For this review, take the finished solid that the model builds, in its own axes (mm). Coordinates: 2 decimals unless noted, no trailing zeros. Write each loop counter-clockwise with the first axis right and the second up, starting at its lowest first coordinate (ties: lowest second). Pieces come first, ordered by that corner, then holes. Notation, with made-up numbers: (62.25, 10.25) -> (94.25, 10.25) arc R30 ccw to (94.25, 41.25) -> close; hole circle Ø7 at (34, 53). An arc over 180 degrees is marked (long way). Put each result on its own line as item: value. Start each with the question number.
Item 1: Consider section B-B on x = -38.5. Give the boundary of the cut face in (y, z).
Item 2: Consider section C-C on y = 65. Give the boundary of the cut face in (x, z), and give its area (3 significant figures).
Item 3: To check wall thickness, follow L1, parallel to Y at x = -39.5, z = 4.5; L2, parallel to Y at x = -122, z = 1.8; L3, parallel to Y at x = -122.5, z = 2.4. State the ranges of each line that lie inside material, in increasing order.
Item 4: Insertion check: P1, Ø1.5, axis at x = -141.5, z = 3.5, coming from the +Y side; P2, Ø1.5, axis at y = 63, z = 1.5, coming from the +X side; P3, Ø1.5, axis at x = -116.5, z = 2, coming from the +Y side. Each pin has a flat end and moves straight along its axis. Give the tip position at first contact, or say it passes through.
Autodesk Inventor part; units mm, degrees
ref_plane "YZ Plane" through (0, 0, 0) normal (1, 0, 0) x (0, 1, 0)
ref_plane "XZ Plane" through (0, 0, 0) normal (0, 1, 0) x (-1, 0, 0)
ref_plane "XY Plane" through (0, 0, 0) normal (0, 0, 1) x (1, 0, 0)
sketch "Sketch1" plane through (0, 0, 0) normal (0, 0, 1) x (1, 0, 0)
  line L0 (0, 0) -> (0, 92)
  line L1 (0, 92) -> (-70, 92)
  line L2 (-70, 92) -> (-161.8477, 0)
  line L3 (-161.8477, 0) -> (0, 0)
  dimension "d1" = 70
  dimension "d2" = 130
  dimension "d7" = 92
extrude "Extrusion1" add sketch "Sketch1" along normal blind 5
sketch "Sketch2" plane through (0, 0, 5) normal (0, 0, 1) x (1, 0, 0)
  line L0 (-70, 92) -> (-161.8477, 0)
  line L1 (-143.5135, 18.3646) -> (-139.9043, 14.7614)
  line L2 (-139.9043, 14.7614) -> (-121.4641, 33.2321)
  line L3 (-121.4641, 33.2321) -> (-125.0733, 36.8354)
  line L4 (-106.7744, 55.1646) -> (-103.1652, 51.5614)
  line L5 (-103.1652, 51.5614) -> (-84.725, 70.0321)
  line L6 (-84.725, 70.0321) -> (-88.3342, 73.6354)
  line L7 (-123.2687, 35.0338) -> (-104.9698, 53.363) construction
  line L8 (-114.1192, 44.1984) -> (-115.9239, 46)
  line L9 (-161.8477, 0) -> (0, 0)
  line L10 (-129.5282, 0) -> (-97.0586, 0)
  line L11 (-97.0586, 0) -> (-97.0586, 5.1)
  line L12 (-97.0586, 5.1) -> (-129.5282, 5.1)
  line L13 (-129.5282, 5.1) -> (-129.5282, 0)
  line L14 (-64.7891, 0) -> (-32.3195, 0)
  line L15 (-32.3195, 0) -> (-32.3195, 5.1)
  line L16 (-32.3195, 5.1) -> (-64.7891, 5.1)
  line L17 (-64.7891, 5.1) -> (-64.7891, 0)
  line L18 (0, 18.35) -> (-5.1, 18.35)
  line L19 (-5.1, 18.35) -> (-5.1, 36.85)
  line L20 (-5.1, 36.85) -> (0, 36.85)
  line L21 (0, 36.85) -> (0, 18.35)
  line L22 (0, 55.15) -> (-5.1, 55.15)
  line L23 (-5.1, 55.15) -> (-5.1, 73.65)
  line L24 (-5.1, 73.65) -> (0, 73.65)
  line L25 (0, 73.65) -> (0, 55.15)
  line L26 (0, 92) -> (-70, 92)
  line L27 (-46.7167, 92) -> (-23.2833, 92)
  line L28 (-23.2833, 92) -> (-23.2833, 86.9)
  line L29 (-23.2833, 86.9) -> (-46.7167, 86.9)
  line L30 (-46.7167, 86.9) -> (-46.7167, 92)
  line L31 (0, 0) -> (0, 92)
  line L32 (-2.55, 36.85) -> (-2.55, 55.15) construction
  line L33 (-64.7891, 2.55) -> (-97.0586, 2.55) construction
  point P0 (-35, 86.9)
  point P1 (-35, 92)
  point P2 (-80.9239, 2.55)
  point P3 (-80.9239, 0)
  point P4 (-2.55, 46)
  point P5 (0, 46)
  point P6 (-35, 92)
  dimension "d8" = 130
  dimension "d9" = 26.1
  dimension "d10" = 25.9
  dimension "d13" = 5.1
  dimension "d14" = 70
  dimension "d15" = 92
  dimension "d16" = 161.8477
  dimension "d17" = 32.2695
  dimension "d18" = 32.4695
  dimension "d19" = 18.3
  dimension "d20" = 18.5
  dimension "d21" = 23.4333
extrude "Extrusion2" cut sketch "Sketch2" against normal blind 10 contours L6 L5 L4 L0 | L26 L28 L29 L30 | L3 L2 L1 L0 | L25 L22 L23 L24 | L21 L18 L19 L20 | L13 L12 L11 L9 | L17 L16 L15 L9
sketch "Sketch3" plane through (0, 0, 5) normal (0, 0, 1) x (1, 0, 0)
  line L0 (-5.1, 36.85) -> (0, 36.85)
  line L1 (0, 36.85) -> (0, 55.15)
  line L2 (0, 55.15) -> (-5.1, 55.15)
  line L3 (-5.1, 55.15) -> (-5.1, 73.65)
  line L4 (-5.1, 73.65) -> (0, 73.65)
  line L5 (0, 73.65) -> (0, 92)
  line L6 (0, 92) -> (-23.2833, 92)
  line L7 (-23.2833, 92) -> (-23.2833, 86.9)
  line L8 (-23.2833, 86.9) -> (-46.7167, 86.9)
  line L9 (-46.7167, 86.9) -> (-46.7167, 92)
  line L10 (-46.7167, 92) -> (-70, 92)
  line L11 (-70, 92) -> (-88.3342, 73.6354)
  line L12 (-88.3342, 73.6354) -> (-84.725, 70.0321)
  line L13 (-84.725, 70.0321) -> (-103.1652, 51.5614)
  line L14 (-103.1652, 51.5614) -> (-106.7744, 55.1646)
  line L15 (-106.7744, 55.1646) -> (-125.0733, 36.8354)
  line L16 (-125.0733, 36.8354) -> (-121.4641, 33.2321)
  line L17 (-121.4641, 33.2321) -> (-139.9043, 14.7614)
  line L18 (-139.9043, 14.7614) -> (-143.5135, 18.3646)
  line L19 (-143.5135, 18.3646) -> (-161.8477, 0)
  line L20 (-161.8477, 0) -> (-129.5282, 0)
  line L21 (-129.5282, 0) -> (-129.5282, 5.1)
  line L22 (-129.5282, 5.1) -> (-97.0586, 5.1)
  line L23 (-97.0586, 5.1) -> (-97.0586, 0)
  line L24 (-97.0586, 0) -> (-64.7891, 0)
  line L25 (-64.7891, 0) -> (-64.7891, 5.1)
  line L26 (-64.7891, 5.1) -> (-32.3195, 5.1)
  line L27 (-32.3195, 5.1) -> (-32.3195, 0)
  line L28 (-32.3195, 0) -> (0, 0)
  line L29 (0, 0) -> (0, 18.35)
  line L30 (0, 18.35) -> (-5.1, 18.35)
  line L31 (-5.1, 18.35) -> (-5.1, 36.85)
  line L32 (-132.1444, 36.8295) -> (-106.7803, 62.2357)
  line L33 (-106.7803, 62.2357) -> (-103.171, 58.6324)
  line L34 (-103.171, 58.6324) -> (-91.796, 70.0263)
  line L35 (-91.796, 70.0263) -> (-95.4053, 73.6295)
  line L36 (-95.4053, 73.6295) -> (-72.0735, 97)
  line L37 (-72.0735, 97) -> (-41.7167, 97)
  line L38 (-41.7167, 97) -> (-41.7167, 91.9)
  line L39 (-41.7167, 91.9) -> (-28.2833, 91.9)
  line L40 (-28.2833, 91.9) -> (-28.2833, 97)
  line L41 (-28.2833, 97) -> (5, 97)
  line L42 (5, 97) -> (5, 68.65)
  line L43 (5, 68.65) -> (-0.1, 68.65)
  line L44 (-0.1, 68.65) -> (-0.1, 60.15)
  line L45 (-0.1, 60.15) -> (5, 60.15)
  line L46 (5, 60.15) -> (5, 31.85)
  line L47 (5, 31.85) -> (-0.1, 31.85)
  line L48 (-0.1, 31.85) -> (-0.1, 23.35)
  line L49 (-0.1, 23.35) -> (5, 23.35)
  line L50 (5, 23.35) -> (5, -5)
  line L51 (5, -5) -> (-37.3195, -5)
  line L52 (-37.3195, -5) -> (-37.3195, 0.1)
  line L53 (-37.3195, 0.1) -> (-59.7891, 0.1)
  line L54 (-59.7891, 0.1) -> (-59.7891, -5)
  line L55 (-59.7891, -5) -> (-102.0586, -5)
  line L56 (-102.0586, -5) -> (-102.0586, 0.1)
  line L57 (-102.0586, 0.1) -> (-124.5282, 0.1)
  line L58 (-124.5282, 0.1) -> (-124.5282, -5)
  line L59 (-124.5282, -5) -> (-173.9046, -5)
  line L60 (-173.9046, -5) -> (-143.5193, 25.4357)
  line L61 (-143.5193, 25.4357) -> (-139.9101, 21.8324)
  line L62 (-139.9101, 21.8324) -> (-128.5351, 33.2263)
  line L63 (-128.5351, 33.2263) -> (-132.1444, 36.8295)
  line L64 (-143.5135, 18.3646) -> (-147.0519, 21.8972)
  line L65 (-161.8477, 0) -> (-168.9129, 0)
  line L66 (-125.0733, 36.8354) -> (-128.6118, 40.368)
  line L67 (-106.7744, 55.1646) -> (-110.3129, 58.6972)
  line L68 (-103.171, 58.6324) -> (-106.7744, 55.1646)
  line L69 (-91.796, 70.0263) -> (-88.3342, 73.6354)
  line L70 (-88.3342, 73.6354) -> (-91.8727, 77.168)
  line L71 (-70, 92) -> (-77.0652, 92)
  line L72 (-139.9101, 21.8324) -> (-143.5135, 18.3646)
  line L73 (-125.0733, 36.8354) -> (-128.5351, 33.2263)
  line L74 (-143.5135, 18.3646) -> (-161.8477, 0)
  line L75 (-161.8477, 0) -> (-165.3862, 3.5326)
  dimension "d22" = 5
extrude "Extrusion3" [suppressed]
sketch "Sketch4" plane through (0, 0, 5) normal (0, 0, 1) x (1, 0, 0)
  line L0 (-5.1, 36.85) -> (0, 36.85)
  line L1 (0, 36.85) -> (0, 55.15)
  line L2 (0, 55.15) -> (-5.1, 55.15)
  line L3 (-5.1, 55.15) -> (-5.1, 73.65)
  line L4 (-5.1, 73.65) -> (0, 73.65)
  line L5 (0, 73.65) -> (0, 92)
  line L6 (0, 92) -> (-23.2833, 92)
  line L7 (-23.2833, 92) -> (-23.2833, 86.9)
  line L8 (-23.2833, 86.9) -> (-46.7167, 86.9)
  line L9 (-46.7167, 86.9) -> (-46.7167, 92)
  line L10 (-46.7167, 92) -> (-70, 92)
  line L11 (-70, 92) -> (-88.3342, 73.6354)
  line L12 (-88.3342, 73.6354) -> (-84.725, 70.0321)
  line L13 (-84.725, 70.0321) -> (-103.1652, 51.5614)
  line L14 (-103.1652, 51.5614) -> (-106.7744, 55.1646)
  line L15 (-106.7744, 55.1646) -> (-125.0733, 36.8354)
  line L16 (-125.0733, 36.8354) -> (-121.4641, 33.2321)
  line L17 (-121.4641, 33.2321) -> (-139.9043, 14.7614)
  line L18 (-139.9043, 14.7614) -> (-143.5135, 18.3646)
  line L19 (-143.5135, 18.3646) -> (-161.8477, 0)
  line L20 (-161.8477, 0) -> (-129.5282, 0)
  line L21 (-129.5282, 0) -> (-129.5282, 5.1)
  line L22 (-129.5282, 5.1) -> (-97.0586, 5.1)
  line L23 (-97.0586, 5.1) -> (-97.0586, 0)
  line L24 (-97.0586, 0) -> (-64.7891, 0)
  line L25 (-64.7891, 0) -> (-64.7891, 5.1)
  line L26 (-64.7891, 5.1) -> (-32.3195, 5.1)
  line L27 (-32.3195, 5.1) -> (-32.3195, 0)
  line L28 (-32.3195, 0) -> (0, 0)
  line L29 (0, 0) -> (0, 18.35)
  line L30 (0, 18.35) -> (-5.1, 18.35)
  line L31 (-5.1, 18.35) -> (-5.1, 36.85)
  line L32 (-143.5135, 18.3646) -> (-161.8477, 0)
  line L33 (-158.3209, 3.5326) -> (-154.7825, 0)
  dimension "d27" = 5
extrude "Extrusion4" cut sketch "Sketch4" against normal through all contours L20 L19 L33
properties part number "SidePlate" material "MDF Medium Density Fiberboard"
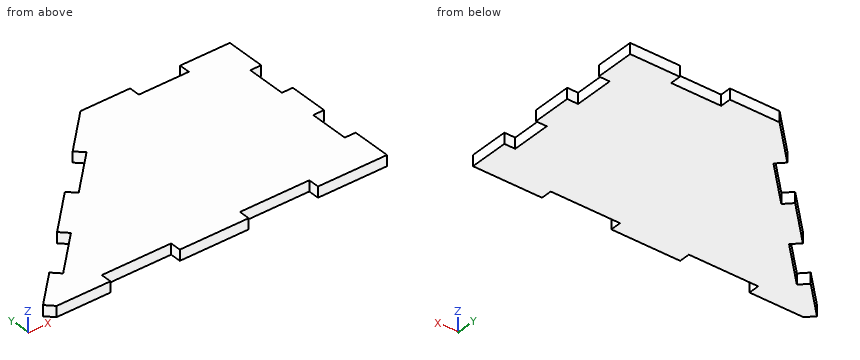
Return value:
1. outline: (5.1, 0) -> (86.9, 0) -> (86.9, 5) -> (5.1, 5) -> close
2. outline: (-89.75, 0) -> (-5.1, 0) -> (-5.1, 5) -> (-89.75, 5) -> close
2. area: 423 mm^2
3. L1: 5.1 to 86.9
3. L2: 5.1 to 32.7, 33.77 to 39.91
3. L3: 5.1 to 32.19, 34.27 to 39.41
4. P1: y = 17.1
4. P2: x = -5.1
4. P3: y = 46.17
